from build123d import *

# Parameters (mm, degrees)
F0_W     = 130
F0_H     = 114
F1_DEPTH = 3
F2_W     = 20
F2_H     = 2.5
F3_DEPTH = 5
F4_R     = 4.99999
F5_R     = 1.5
F6_W     = 4
F6_H     = 7.5
F7_DEPTH = 25


# Not quite as in the source:
# - a fillet or chamfer is up to 0.001 mm smaller than in the source, because OpenCascade refuses the exact size


with BuildPart() as f1:
    # F0 (on Front) → F1 (new body)
    with BuildSketch(Plane.XZ):
        with Locations((65, 57)):
            Rectangle(F0_W, F0_H)
    extrude(amount=F1_DEPTH)

    # F2 (on face) → F3 (join)
    with BuildSketch(Plane.XZ.offset(3)):
        with Locations((10, 112.75)):
            Rectangle(F2_W, F2_H)
        with Locations((120, 112.75)):
            Rectangle(F2_W, F2_H)
    extrude(amount=F3_DEPTH)

    # F4 (radius 5 in the source; OpenCascade refuses exactly that, so slightly less here)
    f4_edges = [f1.edges().sort_by_distance(p)[0] for p in [
        (20, -8, 112.75),
        (110, -8, 112.75),
    ]]
    fillet(f4_edges, radius=F4_R)

    # F5
    f5_edges = [f1.edges().sort_by_distance(p)[0] for p in [
        (7.500005, -8, 114),
        (122.499995, -8, 114),
    ]]
    fillet(f5_edges, radius=F5_R)

    # F6 (on face) → F7 (cut)
    with BuildSketch(Plane(origin=(0, 0, 0), x_dir=(-1, 0, 0), z_dir=(0, 1, 0))):
        with Locations((-2, 3.75)):
            Rectangle(F6_W, F6_H)
    extrude(amount=-F7_DEPTH, mode=Mode.SUBTRACT)


solid = f1.part
For this review, take the finished solid that the model builds, in its own axes (mm). A direction names the side the tool comes from. Round coordinates to 2 decimals unless told otherwise and drop trailing zeros. Loops run counter-clockwise (first coordinate to the right, second up) from the corner with the lowest first, then second, coordinate; pieces in that order, holes last. Notation, with made-up numbers: (19.5, 59) - (61.5, 59) arc R34 cw to (61.5, 90) - close; hole circle Ø2 at (36.5, -32.5). An arc over 180 degrees is marked (long way). One line per item, written item: value. Start each with the question number.
Item 1: Clearance check with flat-ended pins moving along their axes: pin 1 Ø4 at (x, y) = (120, -5.5) entering from -Z; pin 2 Ø1.5 at (x, y) = (1.5, -2) entering from -Z; pin 3 Ø2 at (x, z) = (112.5, 34.5) entering from +Y; pin 4 Ø0.9 at (y, z) = (-1.5, 3.5) entering from -X. State where each tip first meets the part, or that it passes through.
Item 2: The part is to be moulded in two halves that separate along X. For faces 1 (the flat face through (10, -5, 111.5)), 2 (the flat face through (4, -1, 4)), 3 (the cylindrical face through (19, -6, 112)), say which applies: +X half, -X half, draft (parallel to the pull), parting line (faces both ways), or undercut.
Item 3: For L1, parallel to Z at x = 6, y = -3.25; L2, parallel to Y at x = 35, z = 59, list the stretches that pass through material, from the lowest coordinate up.
Item 4: For faces 4 (the flat face through (2, -1, 7.5)), 5 (the flat face through (120, -5, 111.5)), 6 (the cylindrical face through (112, -7, 112)), list the 3-axis set-ups (+Z, -Z, +X, -X, +Y, -Y) from which the entire face can be reached by the end or side of a thin tool; tool diameter is ignored.
Item 5: Take a section at B-B (z = 90.5). Give the boundary of the cut face in (x, y).
Item 6: Take a section at A-A (x = 96.5). Give the boundary of the cut face in (y, z), plus the area to 3 significant figures.
Answer below:
1. pin 1: stops at z = 111.5
1. pin 2: stops at z = 7.5
1. pin 3: stops at y = 0
1. pin 4: stops at x = 4
2. face 1: draft
2. face 2: -X half
2. face 3: undercut
3. L1: z = 111.5 to 114
3. L2: y = -3 to 0
4. face 4: -Z, -X, +Y, -Y
4. face 5: -Z, +X, -X, -Y
4. face 6: +Z, -Z, -Y
5. outline: (0, -3) - (130, -3) - (130, 0) - (0, 0) - close
6. outline: (-3, 0) - (0, 0) - (0, 114) - (-3, 114) - close
6. area: 342 mm2
